Design review of the part built by this model. Coordinates are the model's own, in mm. Face numbers are marked on the shaded views. A direction names the side the tool comes from. Coordinates: 2 decimals unless noted, no trailing zeros. Write each loop counter-clockwise with the first axis right and the second up, starting at its lowest first coordinate (ties: lowest second). Pieces come first, ordered by that corner, then holes. Notation, with made-up numbers: M 63.5,31.5 L 110.5,31.5 A21 ccw 110.5,58.5 Z; hole C 48,28 d9. An arc over 180 degrees is marked long. One line per question, with ' | ' between items.
from build123d import *

# Parameters (mm, degrees)
ESQUISSE1_W             = 26
ESQUISSE1_H             = 26
BOSS_EXTRU_1_DEPTH      = 26.5
ENL_V_MAT_EXTRU_1_DEPTH = 19.5
ESQUISSE4_W             = 11
ESQUISSE4_H             = 10
ENL_V_MAT_EXTRU_2_DEPTH = 40.33509883
ENL_V_MAT_EXTRU_3_DEPTH = 57.098128311
ESQUISSE6_W             = 17
ESQUISSE6_H             = 17
ENL_V_MAT_EXTRU_4_DEPTH = 44.211248008


with BuildPart() as part:
    # Esquisse1 → Boss.-Extru.1 (new, symmetric)
    with BuildSketch(Plane(origin=(0, 0, 0), x_dir=(0, 0, -1), z_dir=(1, 0, 0))):
        Rectangle(ESQUISSE1_W, ESQUISSE1_H)
    extrude(amount=BOSS_EXTRU_1_DEPTH, both=True)

    # Esquisse3 → Enlèv. mat.-Extru.1 (cut, symmetric)
    with BuildSketch(Plane(origin=(0, 0, 0), x_dir=(0, 0, -1), z_dir=(1, 0, 0))):
        Polygon((-13, -13), (8, 13), (-13, 13), align=None)
    extrude(amount=ENL_V_MAT_EXTRU_1_DEPTH, both=True, mode=Mode.SUBTRACT)

    # Esquisse4 → Enlèv. mat.-Extru.2 (cut, through all)
    with BuildSketch(Plane.XY.offset(13)):
        with Locations((21, 13)):
            Rectangle(ESQUISSE4_W, ESQUISSE4_H)
    enl_v_mat_extru_2 = extrude(amount=-ENL_V_MAT_EXTRU_2_DEPTH, mode=Mode.SUBTRACT)

    # Symétrie1: Enlèv. mat.-Extru.2 across plane
    add(enl_v_mat_extru_2.mirror(Plane(origin=(0, 0, 0), x_dir=(0, 0, 1), z_dir=(1, 0, 0))), mode=Mode.SUBTRACT)

    # Esquisse5 → Enlèv. mat.-Extru.3 (cut, through all)
    with BuildSketch(Plane(origin=(26.5, 0, 0), x_dir=(0, 0, -1), z_dir=(1, 0, 0))):
        Polygon((-13, 3.7), (0.488461538, 3.7), (3.961538462, 8), (-13, 8), align=None)
    extrude(amount=-ENL_V_MAT_EXTRU_3_DEPTH, mode=Mode.SUBTRACT)

    # Esquisse6 → Enlèv. mat.-Extru.4 (cut, through all, along a direction that is not the sketch's normal)
    with BuildSketch(Plane(origin=(0, 1.222023277, 1.5129812), x_dir=(1, 0, 0), z_dir=(0, 0.6283371070876215, 0.7779411802037214))):
        with Locations((0, -2.781617735)):
            Rectangle(ESQUISSE6_W, ESQUISSE6_H)
    extrude(amount=-ENL_V_MAT_EXTRU_4_DEPTH, dir=(0, 0, 1), mode=Mode.SUBTRACT)


solid = part.part
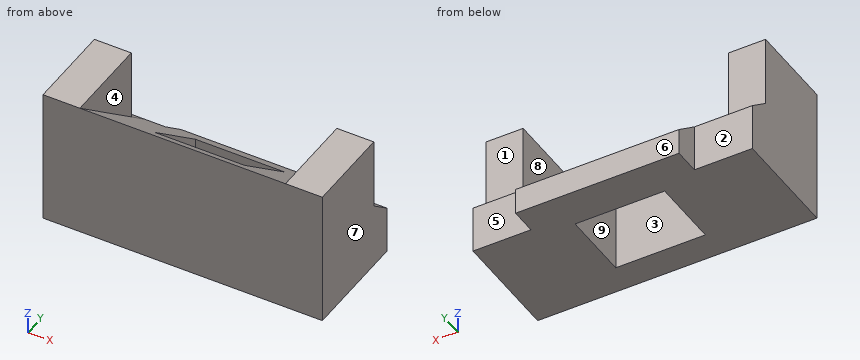
1. Take a section at D-D (x = 22). Write out the cut boundary in (y, z).
Answer sheet:
outline: M -13,-13 L 8,-13 L 8,-3.96 L 3.7,-0.49 L 3.7,13 L -13,13 Z
2. Take a section at B-B (y = -1). Write out the cut boundary in (x, z).
Answer sheet:
outline: M -26.5,-13 L -8.5,-13 L -8.5,3.31 L -19.5,3.31 L -19.5,13 L -26.5,13 Z; M 8.5,-13 L 26.5,-13 L 26.5,13 L 19.5,13 L 19.5,3.31 L 8.5,3.31 Z
3. Tool access review of the marked faces 1, 2, 3, 4 and 5: name each direction out of +Z, -Z, +X, -X, +Y, -Y from which nothing blocks a thin tool from reaching the whole face with its end or side.
Answer sheet:
face 1: +Z, +X, -X, +Y | face 2: +Z, -Z, -X, +Y | face 3: +Z, -Z | face 4: +Z, +Y | face 5: +Z, -Z, +X, +Y
4. Take a section at A-A (x = 5.5). Write out the cut boundary in (y, z).
Answer sheet:
outline: M -13,-13 L -7.55,-13 L -7.55,8.6 L -13,13 Z; M 5.67,-13 L 13,-13 L 13,-8 L 5.67,-2.08 Z
5. Insertion check: pin 1 Ø1 at (x, y) = (-2.5, 7) entering from +Z; pin 2 Ø4 at (y, z) = (11.5, -10) entering from +X; pin 3 Ø12 at (x, y) = (11, -4) entering from +Z. Each pin has a flat end and moves straight along its axis. Give the tip position at first contact, or say it passes through.
Answer sheet:
pin 1: z = -2.75 | pin 2: x = 15.5 | pin 3: z = 10.58
6. Take a section at C-C (z = -10.5). Write out the cut boundary in (x, y).
Answer sheet:
outline: M -26.5,-13 L 26.5,-13 L 26.5,8 L 15.5,8 L 15.5,13 L -15.5,13 L -15.5,8 L -26.5,8 Z; hole M -8.5,-7.55 L 8.5,-7.55 L 8.5,5.67 L -8.5,5.67 Z
7. Draft analysis for pull direction X (two halves, no side actions). For the marked faces 6, 7, 8 and 9, state which applies: pulls with the +X half, pulls with the -X half, needs draft (parallel to the pull), parting line crosses it, or undercut.
Answer sheet:
face 6: needs draft | face 7: pulls with the +X half | face 8: undercut | face 9: undercut
8. To check wall thickness, follow line 1 along X through (y, z) = (-6.5, 7); line 2 along Z through (x, y) = (-11.5, -1.5); line 3 along X through (y, z) = (2.5, 4.75). State the ranges of each line that lie inside material, in increasing order. Write a range as [from, to].
Answer sheet:
line 1: [-26.5, -8.5], [8.5, 26.5] | line 2: [-13, 3.71] | line 3: [-26.5, -19.5], [19.5, 26.5]
